Read the model definition and answer for the solid it produces. Units are mm, in the model's axes. A direction names the side the tool comes from. Coordinates: 2 decimals unless noted, no trailing zeros. Write each loop counter-clockwise with the first axis right and the second up, starting at its lowest first coordinate (ties: lowest second). Pieces come first, ordered by that corner, then holes. Notation, with made-up numbers: (22.25, 34) - (37.25, 34) arc R17 cw to (37.25, 56) - close; hole circle Ø4 at (27, -28.75). An arc over 180 degrees is marked (long way). Return JSON: item names as keys, results as strings.
```python
from build123d import *

# Parameters (mm, degrees)
F3_R      = 6.60593
F3_R_2    = 5.037678
F0_DEPTH  = 8.89
F4_R      = 11.149828
F5_DEPTH  = 2.54
F1_R      = 19.383662
F2_DEPTH  = 4.445
F2_FACE_R = 19.383662
F6_DEPTH  = 4.445


with BuildPart() as f0:
    # F3 (on Top) → F0 (new body)
    with BuildSketch(Plane.XY):
        Circle(F3_R)
        Circle(F3_R_2, mode=Mode.SUBTRACT)
    extrude(amount=F0_DEPTH)

    # F4 (on Top) → F5 (join)
    with BuildSketch(Plane.XY):
        Circle(F4_R)
    extrude(amount=F5_DEPTH)

    # F1 (on Top) → F2 (join)
    with BuildSketch(Plane.XY):
        Circle(F1_R)
    extrude(amount=F2_DEPTH)

    # F2_face (on face) → F6 (join)
    with BuildSketch(Plane(origin=(0, 0, 0), x_dir=(1, 0, 0), z_dir=(0, 0, -1))):
        Circle(F2_FACE_R)
    extrude(amount=F6_DEPTH)


solid = f0.part
```
(1) Determine the mould class of faces 1 (the face through (-0.86, 6.55, 6.64)), 2 (the face through (0, 0, 4.445)), 3 (the face through (0, 0, -4.445)) for opening direction Y: +Y half, -Y half, draft (parallel to the pull), parting line (faces both ways), or undercut.
Answer:
{"face 1": "parting line", "face 2": "undercut", "face 3": "draft"}
(2) A cutting plane is placed at A-A (y = 0). Determine the outline of the cut face in (x, z) (3 decimals).
Answer:
{"outline": "(-19.384, -4.445) - (19.384, -4.445) - (19.384, 4.445) - (6.606, 4.445) - (6.606, 8.89) - (5.038, 8.89) - (5.038, 4.445) - (-5.038, 4.445) - (-5.038, 8.89) - (-6.606, 8.89) - (-6.606, 4.445) - (-19.384, 4.445) - close"}
(3) Flat-ended cylindrical pins translate along their axes: P1, Ø4, axis at x = -12.5, z = -1.5, coming from the +Y side; P2, Ø9, axis at x = 0, y = 0, coming from the +Z side (3 decimals); P3, Ø4, axis at x = -0.5, z = 3, coming from the -Y side. Find the tip coordinate at first contact, or state that the pin passes through.
Answer:
{"P1": "y = 16.29", "P2": "z = 4.445", "P3": "y = -19.38"}
(4) A cutting plane is placed at D-D (z = 0). Determine the outline of the cut face in (x, y), and give its area (3 significant figures).
Answer:
{"outline": "circle Ø38.77 at (0, 0)", "area": "1,180 mm²"}
(5) Straight lines are drawn through the part: line 1 (X direction, y = 0, z = 5.45); line 2 (Y direction, x = 1.5, z = 8.75). For each, find the intervals that lie inside material, in ascending order. Write a range as from..to.
Answer:
{"line 1": "-6.61..-5.04, 5.04..6.61", "line 2": "-6.43..-4.81, 4.81..6.43"}
(6) Which of the six approach directions +Z, -Z, +X, -X, +Y, -Y give full straight-line access (tool end or side, diameter ignored) to faces 4 (the face through (2, -5, 8.89)), 5 (the face through (8, 0, 4.445))?
Answer:
{"face 4": "+Z, +X, -X, +Y, -Y", "face 5": "+Z"}
(7) A cutting plane is placed at C-C (z = 8.25). Determine the outline of the cut face in (x, y), and give its area (3 significant figures).
Answer:
{"outline": "circle Ø13.21 at (0, 0); hole circle Ø10.08 at (0, 0)", "area": "57.4 mm²"}
